Check sheet for the modelled part. Datum: model origin and axes. Units: mm. Coordinates: 2 decimals unless noted, no trailing zeros. Write each loop counter-clockwise with the first axis right and the second up, starting at its lowest first coordinate (ties: lowest second). Pieces come first, ordered by that corner, then holes. Notation, with made-up numbers: M -31.5,2.5 L 18.5,2.5 A26 ccw 18.5,39.5 Z; hole C 37,-24.5 d9. An arc over 180 degrees is marked long. Answer as CSV lines item,"result".
from build123d import *

# Parameters (mm, degrees)
SKETCH1_W               = 300
SKETCH1_H               = 15
BOSS_EXTRUDE1_DEPTH     = 150
SKETCH5_R               = 3.5
CUT_EXTRUDE3_DEPTH      = 1
CUT_EXTRUDE3_DEPTH_BACK = 16
SKETCH8_R               = 2.5
CUT_EXTRUDE5_DEPTH      = 16
FILLET4_R               = 40
SKETCH9_R               = 2.5
CUT_EXTRUDE6_DEPTH      = 16


with BuildPart() as part:
    # Sketch1 → Boss-Extrude1 (new body, symmetric)
    with BuildSketch(Plane.XY):
        Rectangle(SKETCH1_W, SKETCH1_H)
    extrude(amount=BOSS_EXTRUDE1_DEPTH, both=True)

    # Sketch5 → Cut-Extrude3 (cut, two sides)
    with BuildSketch(Plane.XZ.offset(7.5)) as cut_extrude3_sk:
        with Locations((50, 0)):
            Circle(SKETCH5_R)
        with Locations((-50, 0)):
            Circle(SKETCH5_R)
    extrude(amount=CUT_EXTRUDE3_DEPTH, mode=Mode.SUBTRACT)
    extrude(cut_extrude3_sk.sketch, amount=-CUT_EXTRUDE3_DEPTH_BACK, mode=Mode.SUBTRACT)

    # Sketch8 → Cut-Extrude5 (cut, through all)
    with BuildSketch(Plane.XZ.offset(7.5)):
        with Locations((-126.213203436, 83.786796564)):
            Circle(SKETCH8_R)
        with Locations((-83.786796564, 126.213203436)):
            Circle(SKETCH8_R)
        with Locations((126.213203436, 83.786796564)):
            Circle(SKETCH8_R)
        with Locations((83.786796564, 126.213203436)):
            Circle(SKETCH8_R)
        with Locations((83.786796564, -126.213203436)):
            Circle(SKETCH8_R)
        with Locations((126.213203436, -83.786796564)):
            Circle(SKETCH8_R)
        with Locations((-126.213203436, -83.786796564)):
            Circle(SKETCH8_R)
        with Locations((-83.786796564, -126.213203436)):
            Circle(SKETCH8_R)
    extrude(amount=-CUT_EXTRUDE5_DEPTH, mode=Mode.SUBTRACT)

    # Fillet4
    fillet4_edges = [part.edges().sort_by_distance(p)[0] for p in [
        (-150, 0, 150),
        (150, 0, 150),
        (-150, 0, -150),
        (150, 0, -150),
    ]]
    fillet(fillet4_edges, radius=FILLET4_R)

    # Sketch9 → Cut-Extrude6 (cut, through all)
    with BuildSketch(Plane(origin=(0, -7.5, 0), x_dir=(-1, 0, 0), z_dir=(0, -1, 0))):
        with Locations((43, -135)):
            Circle(SKETCH9_R)
        with Locations((-43, -135)):
            Circle(SKETCH9_R)
        with Locations((-43, -95)):
            Circle(SKETCH9_R)
        with Locations((43, -95)):
            Circle(SKETCH9_R)
        with Locations((-43, 95)):
            Circle(SKETCH9_R)
        with Locations((-43, 135)):
            Circle(SKETCH9_R)
        with Locations((43, 135)):
            Circle(SKETCH9_R)
        with Locations((43, 95)):
            Circle(SKETCH9_R)
    extrude(amount=-CUT_EXTRUDE6_DEPTH, mode=Mode.SUBTRACT)


solid = part.part
1) Section check C-C, the plane y = -4.25. Give the number of separate pieces and of enclosed holes in the cut face, plus the area to 3 significant figures.
Answer key:
separate pieces,"1"
enclosed holes,"18"
area,"88,200 mm2"
2) Section check A-A, the plane x = 50. Record the boundary of the cut face in (y, z), plus the area to 4 significant figures.
Answer key:
outline,"M -7.5,-150 L 7.5,-150 L 7.5,-3.5 L -7.5,-3.5 Z; M -7.5,3.5 L 7.5,3.5 L 7.5,150 L -7.5,150 Z"
area,"4,395 mm2"
3) Section check B-B, the plane z = 0. Record the boundary of the cut face in (x, y), plus the area to 3 significant figures.
Answer key:
outline,"M -150,-7.5 L -53.5,-7.5 L -53.5,7.5 L -150,7.5 Z; M -46.5,-7.5 L 46.5,-7.5 L 46.5,7.5 L -46.5,7.5 Z; M 53.5,-7.5 L 150,-7.5 L 150,7.5 L 53.5,7.5 Z"
area,"4,290 mm2"
4) Mould release check, pull along Z, two halves, no side actions. Record for faces 1 (the face through (137.972, 0.105, 138.594)), 2 (the face through (-53.497, -0.105, 0.154)), 3 (the face through (-2, 0, -150)): pulls with the +Z half, pulls with the -Z half, needs draft (parallel to the pull), parting line crosses it, or undercut.
Answer key:
face 1,"pulls with the +Z half"
face 2,"undercut"
face 3,"pulls with the -Z half"
5) Thickness scan on line 1 along X through (y, z) = (3, 95); line 2 along Z through (x, y) = (43, 2.25); line 3 along X through (y, z) = (-3.5, 82.5). Record the ranges inside material, lowest first.
Answer key:
line 1,"x = -150 to -45.5, -40.5 to 40.5, 45.5 to 150"
line 2,"z = -150 to -137.5, -132.5 to -97.5, -92.5 to 92.5, 97.5 to 132.5, 137.5 to 150"
line 3,"x = -150 to -128.36, -124.07 to 124.07, 128.36 to 150"
6) Depth check by flat-ended pin: P1, Ø1.5, axis at x = 111.5, y = -2.5, coming from the -Z side. Enter the tip coordinate at first touch or a pass-through.
Answer key:
P1,"stops at z = -149.99"
